Design review of the part shown in the three views and the two pictorial views. Dimensions are in mm from the part's minimum x, y and z. A direction names the side the tool comes from. Coordinates: 2 decimals unless noted, no trailing zeros. Order: outer loops, then holes, each group sorted by start corner. A loop starts at its lowest first (then second) coordinate and runs counter-clockwise, first axis right, second up. Notation, with made-up numbers: M 40,-34.5 L 70,-34.5 A12 ccw 70,-23.5 Z; hole C 15.25,47 d7. An arc over 180 degrees is marked long. Use CSV: the item, a comma, the result in double quotes.
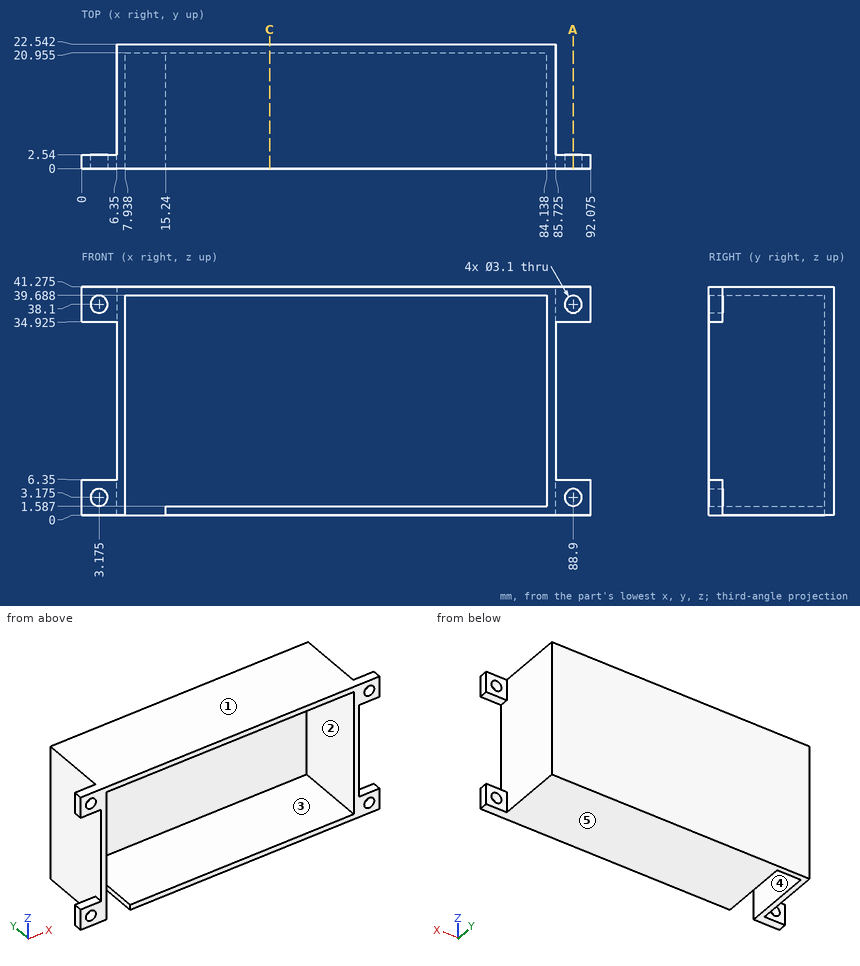
(1) Add section C-C on x = 34. State the section outline as (y, z) points (1 decimal), and give its area (3 significant figures).
The answers:
outline,"M 0,0 L 22.5,0 L 22.5,41.3 L 0,41.3 L 0,39.7 L 21,39.7 L 21,1.6 L 0,1.6 Z"
area,"132 mm2"
(2) Wall thickness on probe 1 along Z at (x, y) = (45.5, 11) (1 decimal); probe 2 along Y at (x, z) = (69, 10.5) (1 decimal); probe 3 along Z at (x, y) = (11.5, 16.25) (1 decimal): over which ranges is each line inside the solid? List them lowest first.
The answers:
probe 1,"z = 0 to 1.6, 39.7 to 41.3"
probe 2,"y = 21 to 22.5"
probe 3,"z = 39.7 to 41.3"
(3) Add section A-A on x = 88.9. Give the number of separate pieces and of enclosed holes in the cut face, and give its area (3 significant figures).
The answers:
separate pieces,"4"
enclosed holes,"0"
area,"16.5 mm2"
(4) The part is to be moulded in two halves that separate along Z. For the marked faces 3, 4 and 5, say which applies: pulls with the +Z half, pulls with the -Z half, needs draft (parallel to the pull), parting line crosses it, or undercut.
The answers:
face 3,"undercut"
face 4,"needs draft"
face 5,"pulls with the -Z half"
(5) Clearance check with flat-ended pins moving along their axes: P1, Ø11.5, axis at y = 16.5, z = 18.5, coming from the -X side; P2, Ø3, axis at y = 5.5, z = 35.5, coming from the -X side; P3, Ø5, axis at x = 14, z = 27, coming from the -Y side (1 decimal); P4, Ø3, axis at x = 88.9, z = 38.1, coming from the +Y side. State where each tip first meets the part, or that it passes through.
The answers:
P1,"stops at x = 6.35"
P2,"stops at x = 6.35"
P3,"stops at y = 21"
P4,"passes through"
(6) For the marked faces 1 and 2, list the 3-axis set-ups (+Z, -Z, +X, -X, +Y, -Y) from which the entire face can be reached by the end or side of a thin tool; tool diameter is ignored.
The answers:
face 1,"+Z, +X, -X, +Y, -Y"
face 2,"-Y"
